Input: part model. Units: mm. Frame: model coordinates. A direction names the side the tool comes from. Coordinates: 2 decimals unless noted, no trailing zeros. Order: outer loops, then holes, each group sorted by start corner. A loop starts at its lowest first (then second) coordinate and runs counter-clockwise, first axis right, second up. Notation, with made-up numbers: (9.25, 66) -> (47.25, 66) arc R36 ccw to (47.25, 101) -> close; hole circle Ø1 at (27, 71). An arc over 180 degrees is marked (long way). One line per item, written item: value. Start each with the question number.
Autodesk Inventor part; units mm, degrees
ref_plane "YZ Plane" through (0, 0, 0) normal (1, 0, 0) x (0, 1, 0)
ref_plane "XZ Plane" through (0, 0, 0) normal (0, 1, 0) x (-1, 0, 0)
ref_plane "XY Plane" through (0, 0, 0) normal (0, 0, 1) x (1, 0, 0)
sketch "TopProfile" plane through (0, 0, 0) normal (0, 0, 1) x (1, 0, 0)
  circle A0 centre (0, 15.5) radius 3.5
  circle A1 centre (0, -15.5) radius 3.5
  line L0 (1.75, 18.5311) -> (-8.5, 24.4489)
  line L1 (-8.5, -23.5511) -> (-8.5, 24.4489)
  arc A2 (1.6248, 12.4) -> (1.6248, -12.4) centre (8.124, 0) ccw
  line L2 (-8.5, -23.5511) -> (-6, -23.5511)
  arc A3 (0.6576, -18.9377) -> (-6, -23.5511) centre (2.5365, -28.7596) ccw
  line L3 (0, -15.5) -> (0, 15.5) construction
  circle A4 centre (0, 15.5) radius 1.5
  circle A5 centre (0, -15.5) radius 1.5
  point P0 (0, 0)
  point P1 (0, 0)
  dimension "d1" = 7
  dimension "d3" = 2.5
  dimension "d4" = 60
  dimension "d5" = 48
  dimension "d6" = 14
  dimension "d7" = 31
  dimension "d9" = 8.5
  dimension "d10" = 3
  dimension "d12" = 10
extrude "TopProfileFeature" add sketch "TopProfile" along normal blind 10
sketch "FrontProfile" plane through (-8.5, -23.5511, 0) normal (0, -1, 0) x (1, 0, 0)
  line L0 (0, 0) -> (0, 10) construction
  line L1 (0, 10) -> (2.5, 10)
  line L2 (12, 0) -> (12, 10) construction
  line L3 (0, 10) -> (12, 10)
  line L4 (12, 10) -> (9.1576, 10)
  line L5 (0, 10) -> (0, 0)
  line L6 (0, 0) -> (2, 0)
  line L7 (2, 0) -> (2, 8)
  line L8 (2, 8) -> (12, 8)
  line L9 (12, 10) -> (12, 8)
  line L10 (0, 0) -> (2.5, 0)
  point P0 (10.1248, 10)
  dimension "d16" = 2
  dimension "d45" = 2
extrude "FrontProfileFeature" cut sketch "FrontProfile" against normal through all keep common part
fillet "SideFilletFeature" radius 1 1 edges at (-8.5, 0.4489, 10)
sketch "Sinks" plane through (0, 0, 10) normal (0, 0, 1) x (1, 0, 0)
  circle A0 centre (0, 15.5) radius 1.5 construction
  circle A1 centre (0, -15.5) radius 1.5 construction
  circle A2 centre (0, 15.5) radius 3.5
  circle A3 centre (0, -15.5) radius 3.5
  line L0 (-1.4875, 18.6682) -> (-7, 21.8509)
  line L1 (-7, 21.8509) -> (-7, 4)
  arc A4 (-1.3472, 12.2697) -> (-6.8509, 4) centre (8.124, 0) ccw
  line L2 (1.75, 18.5311) -> (-7.5, 23.8716) construction
  line L3 (-8.5, 24.4489) -> (-8.5, -23.5511) construction
  arc A5 (1.6248, 12.4) -> (1.6248, -12.4) centre (8.124, 0) ccw construction
  line L4 (-7, -4) -> (-7, -22.3326)
  arc A6 (-6.8509, -4) -> (-1.3472, -12.2697) centre (8.124, 0) ccw
  arc A7 (-2.1532, -18.2593) -> (-7, -22.3326) centre (2.5365, -28.7596) ccw
  arc A8 (0.6576, -18.9377) -> (-6, -23.5511) centre (2.5365, -28.7596) ccw construction
  line L5 (-7, 4) -> (-6.8509, 4)
  line L6 (-6.8509, -4) -> (-7, -4)
  arc A9 (1.6248, 12.4) -> (1.6248, -12.4) centre (8.124, 0) ccw construction
  line L7 (-5.876, 0) -> (-8.5, 0) construction
  line L8 (-8.5, 24.4489) -> (-8.5, -23.5511) construction
  point P0 (0, 0)
  dimension "d20" = 1.5
  dimension "d21" = 1.5
  dimension "d22" = 1.5
  dimension "d23" = 1.5
  dimension "d24" = 1.5
  dimension "d50" = 4
  dimension "d51" = 4
extrude "SinksFeature" cut sketch "Sinks" against normal blind 1 contours A2 A4 L5 L1 L0 | A3 A7 L4 L6 A6
fillet "SinkFilletsFeature" radius 1 10 edges at (-7, 21.8509, 9.5) (-7, 4, 9.5) (-1.3472, 12.2697, 9.5) (-1.4875, 18.6682, 9.5) (-7, -22.3326, 9.5) (-7, -4, 9.5) (-1.3472, -12.2697, 9.5) (-2.1532, -18.2593, 9.5) (-6.8509, 4, 9.5) (-6.8509, -4, 9.5)
sketch "SideHoles" plane through (-8.5, -23.5511, 0) normal (-1, 0, 0) x (0, 0, 1)
  line L0 (10, 0) -> (10, 47.4226) construction
  line L1 (0, 48) -> (9, 48) construction
  circle A0 centre (5, 41.5) radius 1.75
  line L2 (5, 41.5) -> (5, 6.5) construction
  circle A1 centre (5, 24) radius 1.75
  circle A2 centre (5, 6.5) radius 1.75
  line L3 (5, 24) -> (0, 24) construction
  circle A3 centre (5, 15.25) radius 1.75
  circle A4 centre (5, 32.75) radius 1.75
  line L4 (0, 48) -> (0, 0) construction
  line L5 (8, 0) -> (0, 0)
  dimension "d28" = 3.5
  dimension "d30" = 5
  dimension "d33" = 35
  dimension "d43" = 8.75
  dimension "d44" = 8.75
  dimension "d46" = 5
  dimension "d47" = 6.5
  dimension "d48" = 6.5
hole "SideHolesFeature" at (-8.5, 17.9489, 5) at (-8.5, 0.4489, 5) at (-8.5, -17.0511, 5) at (-8.5, 9.1989, 5) at (-8.5, -8.3011, 5) direction (1, 0, 0) diameter 3 end through all
fillet "BottomCornerFilletsFeature" radius 1 2 edges at (-7.5, -23.5511, 0) (-7.5, 23.8716, 0)
equation "\"d21\" = d20"
equation "\"d22\" = d20"
equation "\"d23\" = d20"
equation "\"d24\" = d20"
equation "\"d51\" = d50"
equation "\"d30\" = 0.5 * d29"
equation "\"d43\" = 0.25 * d33"
equation "\"d44\" = d43"
equation "\"d47\" = d48"
properties part number "SpineMiddleCover"
1) Access query for faces 5 (the flat face through (-5.581, 22.764, 8.437)), 6 (the cylindrical face through (-2.795, -18.205, 9.507)). Directions: +Z, -Z, +X, -X, +Y, -Y. A direction counts if a zero-diameter tool reaches every point of the face in a straight line with its end or side. Return the directions, or none.
2) Section query C-C, the plane x = 0. Return the cut outline in (y, z).
3) Ray query, line 1 along Y through (x, z) = (0.25, 8.75); line 2 along X through (y, z) = (-15.5, 9.65); line 3 along Y through (x, z) = (0, 8.8). Return the intervals inside material, ascending. Write a range as from..to.
4) Section query B-B, the plane y = 15.5. Return the cut outline in (x, z).
5) Mould query, pull axis X, two halves, no side actions, for faces 1 (the cylindrical face through (-5.874, -0.213, 8.986)), 2 (the flat face through (-6.1, 0.3, 10)), 3 (the cylindrical face through (-3.5, 15.4, 9.5)), 4 (the cylindrical face through (-2.022, 12.157, 9.507)). Classes: +X half, -X half, draft (parallel to the pull), parting line (faces both ways), or undercut.
6) Section query A-A, the plane z = 5. Return the cut outline in (x, y), plus the area to 3 significant figures.
7) Pin query (flat end, axial travel): pin 1 Ø5 at (y, z) = (17.95, 5) entering from +X; pin 2 Ø3 at (x, z) = (1.5, 7.5) entering from +Y; pin 3 Ø3.5 at (x, y) = (0, 15.5) entering from -Z. Return the tip coordinate at first contact, or that it passes through.
8) Section query D-D, the plane y = 5. Return the cut outline in (x, z).
Entries:
1. face 5: +Z, -Z, +X, +Y
1. face 6: +Z
2. outline: (-19.09, 8) -> (-17, 8) -> (-17, 10) -> (-19.09, 10) -> close; (-14, 8) -> (-11.4, 8) -> (-11.4, 10) -> (-14, 10) -> close; (11.4, 8) -> (14, 8) -> (14, 10) -> (11.4, 10) -> close; (17, 8) -> (19.54, 8) -> (19.54, 10) -> (17, 10) -> close
3. line 1: y = -19.02..-16.98, -14.02..-11.58, 11.58..14.02, 16.98..19.4
3. line 2: x = -8.26..-7, -3.5..-1.5, 1.5..3.5
3. line 3: y = -19.09..-17, -14..-11.4, 11.4..14, 17..19.54
4. outline: (-8.5, 0) -> (-6.5, 0) -> (-6.5, 8) -> (-1.5, 8) -> (-1.5, 10) -> (-3.5, 10) -> (-3.5, 9) -> (-7, 9) -> (-7, 10) -> (-7.5, 10) arc R1 ccw to (-8.5, 9) -> close; (1.5, 8) -> (3.5, 8) -> (3.5, 10) -> (1.5, 10) -> close
5. face 1: +X half
5. face 2: draft
5. face 3: undercut
5. face 4: undercut
6. outline: (-8.5, -23.55) -> (-6.5, -23.55) -> (-6.5, -18.55) -> (-8.5, -18.55) -> close; (-8.5, -15.55) -> (-6.5, -15.55) -> (-6.5, -9.8) -> (-8.5, -9.8) -> close; (-8.5, -6.8) -> (-6.5, -6.8) -> (-6.5, -1.05) -> (-8.5, -1.05) -> close; (-8.5, 1.95) -> (-6.5, 1.95) -> (-6.5, 7.7) -> (-8.5, 7.7) -> close; (-8.5, 10.7) -> (-6.5, 10.7) -> (-6.5, 16.45) -> (-8.5, 16.45) -> close; (-8.5, 19.45) -> (-6.5, 19.45) -> (-6.5, 23.29) -> (-8.5, 24.45) -> close
6. area: 64.8 mm2
7. pin 1: stops at x = -6.5
7. pin 2: stops at y = 19.49
7. pin 3: stops at z = 8
8. outline: (-8.5, 0) -> (-6.5, 0) -> (-6.5, 8) -> (-4.95, 8) -> (-4.95, 10) -> (-7.5, 10) arc R1 ccw to (-8.5, 9) -> close
